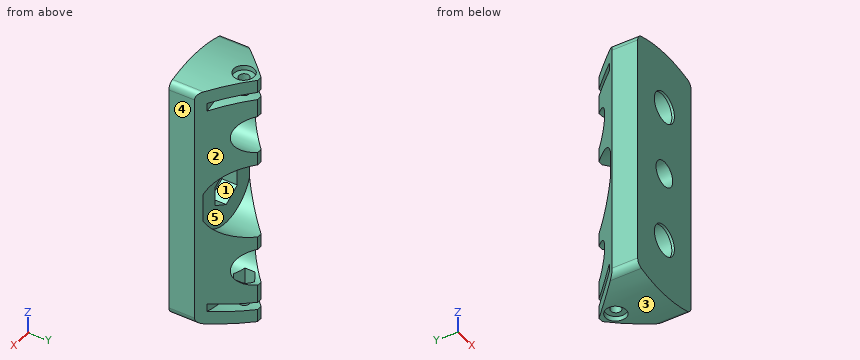
```python
from build123d import *

# Parameters (mm, degrees)
SKETCH1_R               = 5
SKETCH1_R_2             = 6
BOSS_EXTRUDE1_DEPTH     = 25
SKETCH2_R               = 7.5
CUT_EXTRUDE1_DEPTH      = 24
SKETCH3_R               = 15
CUT_EXTRUDE2_DEPTH      = 13
CUT_EXTRUDE3_DEPTH      = 6
SKETCH5_R               = 45
SKETCH5_R_2             = 42
CUT_EXTRUDE_THIN1_DEPTH = 12
CHAMFER1_SIZE           = 15
SKETCH6_R               = 4
CUT_EXTRUDE4_DEPTH      = 2
SKETCH7_R               = 2
CUT_EXTRUDE5_DEPTH      = 20
CUT_EXTRUDE6_REACH      = 111.896
CUT_EXTRUDE6_END_RADIUS = 7.5
CUT_EXTRUDE6_START      = -7.5


with BuildPart() as part:
    # Sketch1 → Boss-Extrude1 (new body)
    with BuildSketch(Plane(origin=(0, 0, 0), x_dir=(1, 0, 0), z_dir=(0, 1, 0))):
        with BuildLine():
            Line((-16, 45.166359163), (-16, -45.166359163))
            ThreePointArc((-16, -45.166359163), (-15.396806386, -46.970609464), (-13.829787234, -48.049318258))
            ThreePointArc((-13.829787234, -48.049318258), (0, -50), (13.829787234, -48.049318258))
            ThreePointArc((13.829787234, -48.049318258), (15.396806386, -46.970609464), (16, -45.166359163))
            Line((16, -45.166359163), (16, 45.166359163))
            ThreePointArc((16, 45.166359163), (15.396806386, 46.970609464), (13.829787234, 48.049318258))
            ThreePointArc((13.829787234, 48.049318258), (0, 50), (-13.829787234, 48.049318258))
            ThreePointArc((-13.829787234, 48.049318258), (-15.396806386, 46.970609464), (-16, 45.166359163))
        make_face()
        with Locations(Location((0, 0, 0), (0, 0, 270))):
            Circle(SKETCH1_R, mode=Mode.SUBTRACT)
        with Locations(Location((0, -27.5, 0), (0, 0, 270))):
            Circle(SKETCH1_R_2, mode=Mode.SUBTRACT)
        with Locations(Location((0, 27.5, 0), (0, 0, 270))):
            Circle(SKETCH1_R_2, mode=Mode.SUBTRACT)
    extrude(amount=BOSS_EXTRUDE1_DEPTH)

    # Sketch2 → Cut-Extrude1 (cut)
    with BuildSketch(Plane(origin=(0, 25, 0), x_dir=(1, 0, 0), z_dir=(0, 1, 0))):
        with Locations(Location((0, 27.5, 0), (0, 0, 270))):
            Circle(SKETCH2_R)
        with Locations(Location((0, -27.5, 0), (0, 0, 270))):
            Circle(SKETCH2_R)
    extrude(amount=-CUT_EXTRUDE1_DEPTH, mode=Mode.SUBTRACT)

    # Sketch3 → Cut-Extrude2 (cut)
    with BuildSketch(Plane(origin=(0, 25, 0), x_dir=(1, 0, 0), z_dir=(0, 1, 0))):
        with Locations(Location((0, 0, 0), (0, 0, 270))):
            Circle(SKETCH3_R)
    extrude(amount=-CUT_EXTRUDE2_DEPTH, mode=Mode.SUBTRACT)

    # Sketch4 → Cut-Extrude3 (cut)
    with BuildSketch(Plane(origin=(0, 12, 0), x_dir=(1, 0, 0), z_dir=(0, 1, 0))):
        Polygon((0, 7.621023553), (-6.6, 3.810511777), (-6.6, -3.810511777), (0, -7.621023553), (6.6, -3.810511777), (6.6, 3.810511777), align=None)
    extrude(amount=-CUT_EXTRUDE3_DEPTH, mode=Mode.SUBTRACT)

    # Sketch5 → Cut-Extrude-Thin1 (cut)
    with BuildSketch(Plane(origin=(0, 25, 0), x_dir=(1, 0, 0), z_dir=(0, 1, 0))):
        Circle(SKETCH5_R)
        Circle(SKETCH5_R_2, mode=Mode.SUBTRACT)
    extrude(amount=-CUT_EXTRUDE_THIN1_DEPTH, mode=Mode.SUBTRACT)

    # Chamfer1
    # the kernel refuses this chamfer: 15 mm, written as the material it takes off along each edge
    with BuildSketch(Plane(origin=(-16, 25, -77.408220497), x_dir=(-0.02749587661058632, -0.9996219169112968, 0), z_dir=(0, 0, 1))) as chamfer1_piece_1:
        Polygon((CHAMFER1_SIZE * 0.999621916911, CHAMFER1_SIZE * 0.0274958766106), (-CHAMFER1_SIZE * 0.0274958766106, CHAMFER1_SIZE * 0.999621916911), (0, 0), align=None)
    extrude(amount=154.816440995, mode=Mode.SUBTRACT)
    with BuildSketch(Plane(origin=(16, 25, 77.408220497), x_dir=(-0.9996219169112968, 0.02749587661058632, 0), z_dir=(0, 0, -1))) as chamfer1_piece_2:
        Polygon((CHAMFER1_SIZE * 0.999621916911, -CHAMFER1_SIZE * 0.0274958766106), (-CHAMFER1_SIZE * 0.0274958766106, -CHAMFER1_SIZE * 0.999621916911), (0, 0), align=None)
    extrude(amount=154.816440995, mode=Mode.SUBTRACT)

    # Sketch6 → Cut-Extrude4 (cut)
    with BuildSketch(Plane.XY.offset(50)):
        with Locations((0, 19)):
            Circle(SKETCH6_R)
    cut_extrude4 = extrude(amount=-CUT_EXTRUDE4_DEPTH, mode=Mode.SUBTRACT)

    # Sketch7 → Cut-Extrude5 (cut)
    with BuildSketch(Plane.XY.offset(48)):
        with Locations((0, 19)):
            Circle(SKETCH7_R)
    cut_extrude5 = extrude(amount=-CUT_EXTRUDE5_DEPTH, mode=Mode.SUBTRACT)

    # Cut-Extrude6: up to this cylinder (the profile starts outside it)
    cut_extrude6_end = Plane(origin=(0, 19, 27.5), z_dir=(0, 1, 0)) * Cylinder(CUT_EXTRUDE6_END_RADIUS, 239.792, mode=Mode.PRIVATE)
    # Sketch8 → Cut-Extrude6 (cut, up to the surface)
    with BuildSketch(Plane.XY.offset(48).offset(CUT_EXTRUDE6_START), mode=Mode.PRIVATE) as cut_extrude6_sk1:
        Polygon((0, 14.900813089), (3.55, 16.950406544), (3.55, 21.049593456), (0, 23.099186911), (-3.55, 21.049593456), (-3.55, 16.950406544), align=None)
    cut_extrude6_tool1 = extrude(cut_extrude6_sk1.sketch, amount=-CUT_EXTRUDE6_REACH, mode=Mode.PRIVATE) - cut_extrude6_end
    cut_extrude6 = cut_extrude6_tool1.solids().sort_by_distance((0, 19, 40.5))[0]
    add(cut_extrude6, mode=Mode.SUBTRACT)

    # Mirror1: Cut-Extrude4, Cut-Extrude5, Cut-Extrude6 across plane
    add(cut_extrude4.mirror(Plane.XY), mode=Mode.SUBTRACT)
    add(cut_extrude5.mirror(Plane.XY), mode=Mode.SUBTRACT)
    add(cut_extrude6.mirror(Plane.XY), mode=Mode.SUBTRACT)


solid = part.part
```
Verification items for the finished model (mm, model axes). Face numbers are marked on the shaded views. A direction names the side the tool comes from. Coordinates: 2 decimals unless noted, no trailing zeros. Loops run counter-clockwise (first coordinate to the right, second up) from the corner with the lowest first, then second, coordinate; pieces in that order, holes last. Notation, with made-up numbers: (43, -14) - (95, -14) arc R17 ccw to (95, -6) - close; hole circle Ø5 at (24.25, 5). An arc over 180 degrees is marked (long way). Answer as a JSON object with one key per item and string values.
(1) Go/stop test with flat-tipped pins: pin 1 Ø6.5 at (x, y) = (0, 19) entering from -Z; pin 2 Ø2 at (x, y) = (-2, 7) entering from +Z; pin 3 Ø14 at (x, z) = (0, -27.5) entering from +Y; pin 4 Ø12 at (x, z) = (0.5, 26) entering from +Y. Record where each tip stops, or that it passes through.
Response:
{"pin 1": "stops at z = -48", "pin 2": "stops at z = 49.99", "pin 3": "stops at y = 1", "pin 4": "stops at y = 25"}
(2) Cross-section at C-C, the plane z = 0. Record the boundary of the cut face in (x, y), then the cut area to 3 significant figures.
Response:
{"outline": "(-16, 0) - (-5, 0) - (-5, 6) - (-6.6, 6) - (-6.6, 12) - (-14, 12) - (-16, 10) - close; (5, 0) - (16, 0) - (16, 10) - (14, 12) - (6.6, 12) - (6.6, 6) - (5, 6) - close", "area": "241 mm²"}
(3) Access from +Z, -Z, +X, -X, +Y, -Y to the whole of each face (thin tool, end or side, straight path). Record for the marked faces 4 and 5.
Response:
{"face 4": "+Z, -Z, +X, +Y, -Y", "face 5": "+Y"}
(4) Cross-section at D-D, the plane z = -12. Record the boundary of the cut face in (x, y), then the cut area to 3 significant figures.
Response:
{"outline": "(-16, 0) - (16, 0) - (16, 10) - (9, 17) - (9, 12) - (-9, 12) - (-9, 17) - (-16, 10) - close", "area": "405 mm²"}
(5) Scan lines: line 1 along Z through (x, y) = (1, 15); line 2 along Z through (x, y) = (0, 0.75); line 3 along Z through (x, y) = (0, 13.5). Record each from-to range of solid material in increasing order.
Response:
{"line 1": "z = -49.99 to -44.99, -41.99 to -34.93, -20.07 to -14.97, 14.97 to 20.07, 34.93 to 41.99, 44.99 to 49.99", "line 2": "z = -50 to -33.5, -21.5 to -5, 5 to 21.5, 33.5 to 50", "line 3": "z = -50 to -45, -42 to -35, -20 to -15, 15 to 20, 35 to 42, 45 to 50"}
(6) Mould release check, pull along Z, two halves, no side actions. Record for the marked faces 1, 2 and 3: pulls with the +Z half, pulls with the -Z half, needs draft (parallel to the pull), parting line crosses it, or undercut.
Response:
{"face 1": "undercut", "face 2": "needs draft", "face 3": "pulls with the -Z half"}
(7) Cross-section at B-B, the plane y = 7. Record the boundary of the cut face in (x, z), then the cut area to 3 significant figures.
Response:
{"outline": "(-16, -45.17) arc R3 ccw to (-13.83, -48.05) arc R50 ccw to (13.83, -48.05) arc R3 ccw to (16, -45.17) - (16, 45.17) arc R3 ccw to (13.83, 48.05) arc R50 ccw to (-13.83, 48.05) arc R3 ccw to (-16, 45.17) - close; hole circle Ø15 at (0, -27.5); hole circle Ø15 at (0, 27.5); hole (-6.6, -3.81) - (0, -7.62) - (6.6, -3.81) - (6.6, 3.81) - (0, 7.62) - (-6.6, 3.81) - close", "area": "2,640 mm²"}
(8) Cross-section at A-A, the plane z = -27.5. Record the boundary of the cut face in (x, y).
Response:
{"outline": "(-16, 0) - (-6, 0) - (-6, 1) - (-7.5, 1) - (-7.5, 18.5) - (-16, 10) - close; (6, 0) - (16, 0) - (16, 10) - (7.5, 18.5) - (7.5, 1) - (6, 1) - close"}
